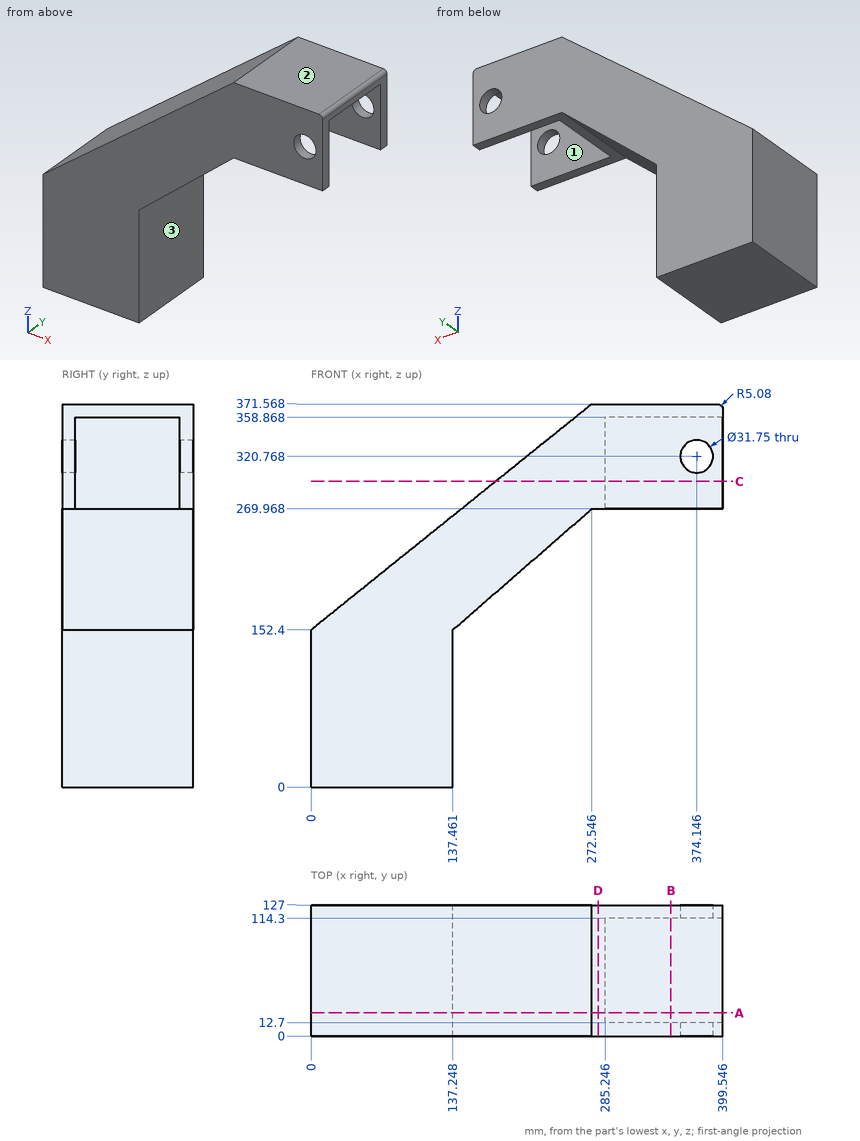
Here's the drawing with two shaded views (mm, measured from the low corner). I have some questions. A direction names the side the tool comes from. Round coordinates to 2 decimals unless told otherwise and drop trailing zeros. Order: outer loops, then holes, each group sorted by start corner. A loop starts at its lowest first (then second) coordinate and runs counter-clockwise, first axis right, second up. Notation, with made-up numbers: M -34,-4 L 13,-4 A25 ccw 13,31 Z; hole C -34.75,40 d4. An arc over 180 degrees is marked long. Use CSV: the item, a comma, the result in double quotes.
1) On a 3-axis mill with a long thin cutter (end or side, diameter ignored), from which of +Z, -Z, +X, -X, +Y, -Y can I reach the whole of each face in a straight line? I mean the marked faces 1, 2 and 3. Say none if no direction works.
Taken from the geometry:
face 1,"-Z, +X"
face 2,"+Z, +X, -X, +Y, -Y"
face 3,"-Z, +X, +Y, -Y"
2) I want a section at A-A (y = 22.5). List the corners of the cut face in (x, z) for me.
Taken from the geometry:
outline,"M 0,0 L 137.25,0 L 137.25,152.4 L 137.46,152.4 L 272.55,269.97 L 285.25,269.97 L 285.25,358.87 L 399.55,358.87 L 399.55,366.49 A5.08 ccw 394.47,371.57 L 272.55,371.57 L 0,152.4 Z"
3) I want a section at C-C (z = 296.5). List the corners of the cut face in (x, y) for me (1 decimal), then the cut area to 3 significant figures.
Taken from the geometry:
outline,"M 179.2,0 L 399.5,0 L 399.5,12.7 L 285.2,12.7 L 285.2,114.3 L 399.5,114.3 L 399.5,127 L 179.2,127 Z"
area,"16,400 mm^2"
4) I want a section at B-B (x = 349). List the corners of the cut face in (y, z) for me, then the cut area to 3 significant figures.
Taken from the geometry:
outline,"M 0,269.97 L 12.7,269.97 L 12.7,358.87 L 114.3,358.87 L 114.3,269.97 L 127,269.97 L 127,371.57 L 0,371.57 Z"
area,"3,870 mm^2"
5) I'm going to push flat-ended pins straight in: P1, Ø3, axis at x = 78, y = 80, coming from the -Z side; P2, Ø6, axis at x = 205.5, y = 19, coming from the -Z side (1 decimal); P3, Ø1.5, axis at y = 42.5, z = 247.5, coming from the +X side. Where does each tip first touch, or does it pass through?
Taken from the geometry:
P1,"z = 0"
P2,"z = 209"
P3,"x = 247.59"
6) I want a section at D-D (x = 278.5). List the corners of the cut face in (y, z) for me, then the cut area to 3 significant figures.
Taken from the geometry:
outline,"M 0,269.97 L 127,269.97 L 127,371.57 L 0,371.57 Z"
area,"12,900 mm^2"
7) I need wall thicknesses on line 1 along X through (y, z) = (105.5, 35.5); line 2 along X through (y, z) = (111.5, 209.5) (1 decimal); line 3 along Z through (x, y) = (76.5, 108.5). Which ranges of each line are inside material? Lowest first, please. Write a range as [from, to].
Taken from the geometry:
line 1,"[0, 137.25]"
line 2,"[71, 203.1]"
line 3,"[0, 213.92]"
